Verification items for the finished model (mm, model axes). A direction names the side the tool comes from. Round coordinates to 2 decimals unless told otherwise and drop trailing zeros. Write each loop counter-clockwise with the first axis right and the second up, starting at its lowest first coordinate (ties: lowest second). Pieces come first, ordered by that corner, then holes. Notation, with made-up numbers: (8.5, 39) -> (53.5, 39) arc R20 cw to (53.5, 60) -> close; hole circle Ø7 at (-16.5, -35.75). An arc over 180 degrees is marked (long way). Use CSV: the item, a comma, the result in double quotes.
```python
from build123d import *

# Parameters (mm, degrees)
SKETCH_1_W          = 170
SKETCH_1_H          = 40
EXTRUDE_1_DEPTH     = 5
EXTRUDE_2_DEPTH     = 5
FILLET_1_R          = 30
SKETCH_3_W          = 5
SKETCH_3_H          = 15
CUT_EXTRUDE_1_DEPTH = 10


with BuildPart() as part:
    # 스케치1 → 보스-돌출1 (new body)
    with BuildSketch(Plane(origin=(0, 0, 0), x_dir=(1, 0, 0), z_dir=(0, 1, 0))):
        with Locations((85, 20)):
            Rectangle(SKETCH_1_W, SKETCH_1_H)
    extrude(amount=EXTRUDE_1_DEPTH)

    # 스케치2 → 보스-돌출2 (add)
    with BuildSketch(Plane(origin=(0, 5, 0), x_dir=(1, 0, 0), z_dir=(0, 1, 0))):
        Polygon((170, 40), (170, 60), (120, 40), align=None)
        Polygon((0, 40), (0, 60), (50, 40), align=None)
    extrude(amount=-EXTRUDE_2_DEPTH)

    # 필렛1
    fillet_1_edges = [part.edges().sort_by_distance(p)[0] for p in [
        (120, 2.5, -40),
        (50, 2.5, -40),
    ]]
    fillet(fillet_1_edges, radius=FILLET_1_R)

    # 스케치3 → 컷-돌출1 (cut)
    with BuildSketch(Plane(origin=(0, 0, 0), x_dir=(-1, 0, 0), z_dir=(0, -1, 0))):
        with Locations((-2.5, 52.5)):
            Rectangle(SKETCH_3_W, SKETCH_3_H)
        with Locations((-2.5, 7.5)):
            Rectangle(SKETCH_3_W, SKETCH_3_H)
        with Locations((-167.5, 52.5)):
            Rectangle(SKETCH_3_W, SKETCH_3_H)
        with Locations((-167.5, 7.5)):
            Rectangle(SKETCH_3_W, SKETCH_3_H)
    extrude(amount=-CUT_EXTRUDE_1_DEPTH, mode=Mode.SUBTRACT)


solid = part.part
```
Q1. Go/stop test with flat-tipped pins: P1, Ø1.5, axis at y = 3.5, z = -5, coming from the +X side; P2, Ø2, axis at x = 136.5, y = 4, coming from the -Z side; P3, Ø1.5, axis at x = 168.5, y = 3, coming from the +Z side. Record where each tip stops, or that it passes through.
Filled in:
P1,"x = 165"
P2,"z = -47"
P3,"z = -15"
Q2. Section check B-B (y = 0.8). Record the cut outline in (x, z).
Filled in:
outline,"(0, -45) -> (5, -45) -> (5, -58) -> (44.64, -42.15) arc R30 cw to (55.78, -40) -> (114.22, -40) arc R30 cw to (125.36, -42.15) -> (165, -58) -> (165, -45) -> (170, -45) -> (170, -15) -> (165, -15) -> (165, 0) -> (5, 0) -> (5, -15) -> (0, -15) -> close"
Q3. Section check C-C (x = 156). Record the cut outline in (y, z), plus the area to 3 significant figures.
Filled in:
outline,"(0, -54.4) -> (5, -54.4) -> (5, 0) -> (0, 0) -> close"
area,"272 mm²"
Q4. Section check D-D (z = -7). Record the cut outline in (x, y).
Filled in:
outline,"(5, 0) -> (165, 0) -> (165, 5) -> (5, 5) -> close"
Q5. Section check A-A (z = -53.5). Record the cut outline in (x, y).
Filled in:
outline,"(5, 0) -> (16.25, 0) -> (16.25, 5) -> (5, 5) -> close; (153.75, 0) -> (165, 0) -> (165, 5) -> (153.75, 5) -> close"
Q6. Material ranges on L1, parallel to Z at x = 113, y = 1.55; L2, parallel to X at y = 3.2, z = -5.5; L3, parallel to Z at x = 129, y = 2.95, recorded low to high.
Filled in:
L1,"-40 to 0"
L2,"5 to 165"
L3,"-43.6 to 0"
Q7. Access from +Z, -Z, +X, -X, +Y, -Y to the whole of each face (thin tool, end or side, straight path). Record for faces 1 (the flat face through (3, 2, -15)), 2 (the flat face through (5, 2, -51)), 3 (the flat face through (168, 2, -15)), 4 (the flat face through (25, 3, -50)).
Filled in:
face 1,"+Z, -X, +Y, -Y"
face 2,"-Z, -X, +Y, -Y"
face 3,"+Z, +X, +Y, -Y"
face 4,"-Z, +Y, -Y"
